from build123d import *

# Parameters (mm, degrees)
EXTRUDE_THIN1_DEPTH = 12


with BuildPart() as part:
    # Sketch1 → Extrude-Thin1 (new body)
    with BuildSketch(Plane.XY):
        with BuildLine():
            Line((20.881, -364.8), (10.881, -364.8))
            ThreePointArc((10.881, -364.8), (8.052572875, -363.628427125), (6.881, -360.8))
            Line((6.881, -360.8), (6.881, 0))
            ThreePointArc((6.881, 0), (0, 6.881), (-6.881, 0))
            Line((-6.881, 0), (-6.881, -425))
            ThreePointArc((-6.881, -425), (0, -431.881), (6.881, -425))
            Line((6.881, -425), (6.881, -380.8))
            ThreePointArc((6.881, -380.8), (8.052572875, -377.971572875), (10.881, -376.8))
            Line((10.881, -376.8), (20.881, -376.8))
            Line((20.881, -376.8), (20.881, -375.28))
            Line((20.881, -375.28), (10.881, -375.28))
            ThreePointArc((10.881, -375.28), (6.977770568, -376.896770568), (5.361, -380.8))
            Line((5.361, -380.8), (5.361, -425))
            ThreePointArc((5.361, -425), (0, -430.361), (-5.361, -425))
            Line((-5.361, -425), (-5.361, 0))
            ThreePointArc((-5.361, 0), (0, 5.361), (5.361, 0))
            Line((5.361, 0), (5.361, -360.8))
            ThreePointArc((5.361, -360.8), (6.977770568, -364.703229432), (10.881, -366.32))
            Line((10.881, -366.32), (20.881, -366.32))
            Line((20.881, -366.32), (20.881, -364.8))
        make_face()
    extrude(amount=EXTRUDE_THIN1_DEPTH)


solid = part.part
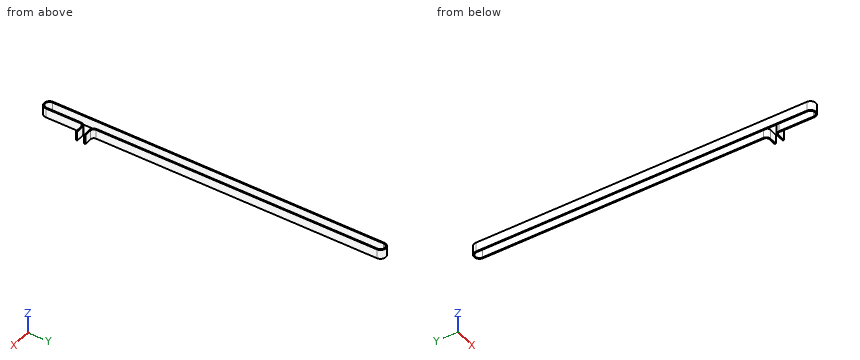
Source: CAD feature listing. Evaluate the final solid. Frame: model axes, mm. Give positions to 0.01 mm unless a question says otherwise; leave off trailing zeros. Write each loop counter-clockwise with the first axis right and the second up, starting at its lowest first coordinate (ties: lowest second). Pieces come first, ordered by that corner, then holes. Notation, with made-up numbers: M 58.5,20 L 82.5,20 A13 cw 82.5,31 Z; hole C 13.5,45 d11. An arc over 180 degrees is marked long. Return JSON: item names as keys, results as strings. Group by question number.
1) First-contact query: pin 1 Ø3 at (x, z) = (9, 10) entering from +Y; pin 2 Ø6 at (x, z) = (18, 1.5) entering from +Y; pin 3 Ø5 at (x, z) = (4.5, 7.5) entering from +Y; pin 4 Ø8 at (x, y) = (11, -47) entering from -Z. Flat tips, straight axial feed; report the tip coordinate or a pass-through.
2) Cut plane C-C, the plane z = 9. Output: boundary loops of the cut face in (x, y).
3) Cut plane A-A, the plane x = 0. Output: boundary loops of the cut face in (y, z).
4) Ray query, L1, parallel to X at y = -161.5, z = 5.5; L2, parallel to Y at x = 18, z = 6; L3, parallel to Y at x = 8, z = 1.75. Return the intervals inside material, ascending.
5) Cut plane B-B, the plane y = -330. Output: boundary loops of the cut face in (x, z).
Data:
{
 "1": {"pin 1": "stops at y = -362.94", "pin 2": "stops at y = -364.8", "pin 3": "stops at y = 6.58", "pin 4": "passes through"},
 "2": {"outline": "M -6.88,-425 A6.88 ccw 6.88,-425 L 6.88,-380.8 A4 cw 10.88,-376.8 L 20.88,-376.8 L 20.88,-375.28 L 10.88,-375.28 A5.52 ccw 5.36,-380.8 L 5.36,-425 A5.36 cw -5.36,-425 L -5.36,0 A5.36 cw 5.36,0 L 5.36,-360.8 A5.52 ccw 10.88,-366.32 L 20.88,-366.32 L 20.88,-364.8 L 10.88,-364.8 A4 cw 6.88,-360.8 L 6.88,0 A6.88 ccw -6.88,0 Z"},
 "3": {"outline": "M -431.88,0 L -430.36,0 L -430.36,12 L -431.88,12 Z; M 5.36,0 L 6.88,0 L 6.88,12 L 5.36,12 Z"},
 "4": {"L1": "x = -6.88 to -5.36, 5.36 to 6.88", "L2": "y = -376.8 to -375.28, -366.32 to -364.8", "L3": "y = -378.03 to -376.09, -365.51 to -363.57"},
 "5": {"outline": "M -6.88,0 L -5.36,0 L -5.36,12 L -6.88,12 Z; M 5.36,0 L 6.88,0 L 6.88,12 L 5.36,12 Z"}
}
